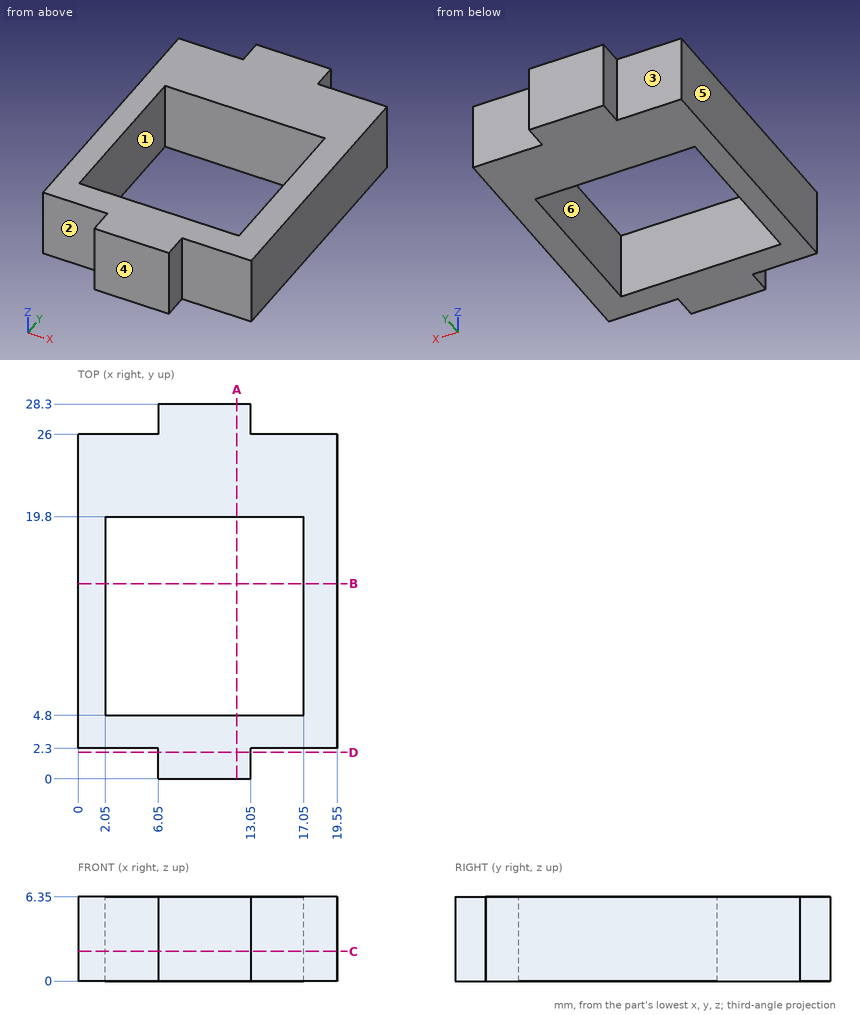
Could you check a few things on this drawing? It's one solid part, dimensions in mm from its lowest x, y, z. A direction names the side the tool comes from. Round coordinates to 2 decimals unless told otherwise and drop trailing zeros. Write each loop counter-clockwise with the first axis right and the second up, starting at its lowest first coordinate (ties: lowest second). Pieces come first, ordered by that corner, then holes. Notation, with made-up numbers: (-16.75, 73.5) -> (8.25, 73.5) arc R3 ccw to (8.25, 78.5) -> close; hole circle Ø9 at (59, -3.5). An arc over 180 degrees is marked (long way). One line per item, written item: value.
1) Suppose I cut it at A-A on x = 12. List the corners of the cut face in (y, z) for me.
Filled sheet:
outline: (0, 0) -> (4.8, 0) -> (4.8, 6.35) -> (0, 6.35) -> close; (19.8, 0) -> (28.3, 0) -> (28.3, 6.35) -> (19.8, 6.35) -> close
2) I'm going to push flat-ended pins straight in: pin 1 Ø1.2 at (y, z) = (27.5, 4.5) entering from -X; pin 2 Ø1 at (x, z) = (3.5, 1) entering from +Y; pin 3 Ø10 at (x, y) = (7, 8.5) entering from -Z; pin 4 Ø1.5 at (x, y) = (3.5, 13.5) entering from +Z. Where does each tip first touch, or does it pass through?
Filled sheet:
pin 1: stops at x = 6.05
pin 2: stops at y = 26
pin 3: stops at z = 0
pin 4: passes through
3) We'd pull the mould along X, two halves only. Please class the marked faces 4, 5 and 6: released by +X, released by -X, zero draft, split by the parting line, or undercut.
Filled sheet:
face 4: zero draft
face 5: released by -X
face 6: undercut
4) Suppose I cut it at C-C on z = 2.25. List the corners of the cut face in (x, y) for me, plus the area to 3 significant figures.
Filled sheet:
outline: (0, 2.3) -> (6.05, 2.3) -> (6.05, 0) -> (13.05, 0) -> (13.05, 2.3) -> (19.55, 2.3) -> (19.55, 26) -> (13.05, 26) -> (13.05, 28.3) -> (6.05, 28.3) -> (6.05, 26) -> (0, 26) -> close; hole (2.05, 4.8) -> (17.05, 4.8) -> (17.05, 19.8) -> (2.05, 19.8) -> close
area: 271 mm2
5) Suppose I cut it at B-B on y = 14.75. List the corners of the cut face in (x, z) for me.
Filled sheet:
outline: (0, 0) -> (2.05, 0) -> (2.05, 6.35) -> (0, 6.35) -> close; (17.05, 0) -> (19.55, 0) -> (19.55, 6.35) -> (17.05, 6.35) -> close
6) If I drill on line 1 (Y direction, x = 3.5, z = 2.5); line 2 (Y direction, x = 9, z = 6); line 3 (X direction, y = 6.5, z = 0.5), over which ranges is the centre line in solid material (lowest first)? Write a range as [from, to].
Filled sheet:
line 1: y = [2.3, 4.8], [19.8, 26]
line 2: y = [0, 4.8], [19.8, 28.3]
line 3: x = [0, 2.05], [17.05, 19.55]
7) For the marked faces 1, 2 and 3, which set-ups out of +Z, -Z, +X, -X, +Y, -Y let a thin tool reach every point of the face, with its end or its side?
Filled sheet:
face 1: +Z, -Z
face 2: +Z, -Z, -X, -Y
face 3: +Z, -Z, -X, +Y
8) Suppose I cut it at D-D on y = 2. List the corners of the cut face in (x, z) for me, plus the area to 4 significant figures.
Filled sheet:
outline: (6.05, 0) -> (13.05, 0) -> (13.05, 6.35) -> (6.05, 6.35) -> close
area: 44.45 mm2
